from build123d import *

# Parameters (mm, degrees)
BOSS_EXTRUDE1_DEPTH = 25.1714


with BuildPart() as part:
    # Sketch1 → Boss-Extrude1 (new body)
    with BuildSketch(Plane.XY.offset(12.5857)):
        with BuildLine():
            Line((-15.096819971, 70.27139515), (-15.096819971, -8.74510913))
            ThreePointArc((-15.096819971, -8.74510913), (-13.34429465, -12.976079529), (-9.113324251, -14.72860485))
            Line((-9.113324251, -14.72860485), (9.113324251, -14.72860485))
            ThreePointArc((9.113324251, -14.72860485), (13.34429465, -12.976079529), (15.096819971, -8.74510913))
            Line((15.096819971, -8.74510913), (15.096819971, 70.27139515))
            Line((15.096819971, 70.27139515), (-15.096819971, 70.27139515))
        make_face()
    extrude(amount=-BOSS_EXTRUDE1_DEPTH)

    # Sketch2 → Revolve1 (revolve)
    with BuildSketch(Plane(origin=(0, 0, 0), x_dir=(1, 0, 0), z_dir=(0, 1, 0))):
        with BuildLine():
            Line((15.767676296, 28.0797), (0.740743286, 28.0797))
            Line((0.740743286, 28.0797), (0.740743286, 12.5857))
            Line((0.740743286, 12.5857), (10.306676296, 12.5857))
            Line((10.306676296, 12.5857), (10.306676296, 23.56842946))
            Line((10.306676296, 23.56842946), (14.543986539, 24.703813318))
            ThreePointArc((14.543986539, 24.703813318), (15.426502661, 25.293491738), (15.767676296, 26.298556857))
            Line((15.767676296, 26.298556857), (15.767676296, 28.0797))
        make_face()
    revolve(axis=Axis((0.740743286, 0, -28.0797), (0, 0, 1)))

    # Sketch3 → Revolve2 (revolve)
    with BuildSketch(Plane(origin=(0, 0, 0), x_dir=(1, 0, 0), z_dir=(0, 1, 0))):
        with BuildLine():
            Line((9.525, -12.5857), (0, -12.5857))
            Line((0, -12.5857), (0, -28.0797))
            Line((0, -28.0797), (14.986, -28.0797))
            Line((14.986, -28.0797), (14.986, -26.20110633))
            ThreePointArc((14.986, -26.20110633), (14.671070491, -25.273353912), (13.856440225, -24.72903537))
            Line((13.856440225, -24.72903537), (9.525, -23.56842946))
            Line((9.525, -23.56842946), (9.525, -12.5857))
        make_face()
    revolve(axis=Axis((0, 0, 3.0607), (0, 0, 1)))

    # Sketch4 → Cut-Revolve1 (revolve, cut)
    with BuildSketch(Plane.XZ):
        Polygon((8.636, 37.6047), (0, 37.6047), (0, -37.6047), (8.636, -37.6047), (8.636, -35.0647), (7.9375, -35.0647), (7.9375, 35.0647), (8.636, 35.0647), align=None)
    revolve(axis=Axis((0, 0, 37.6047), (0, 0, -1)), mode=Mode.SUBTRACT)


solid = part.part
Design review of the part built by this model. Coordinates are the model's own, in mm. A direction names the side the tool comes from. Round coordinates to 2 decimals unless told otherwise and drop trailing zeros. Loops run counter-clockwise (first coordinate to the right, second up) from the corner with the lowest first, then second, coordinate; pieces in that order, holes last. Notation, with made-up numbers: (-29, 59.5) -> (-23, 59.5) arc R18 cw to (-23, 80.5) -> close; hole circle Ø2 at (16, 19). An arc over 180 degrees is marked (long way). Use one line per item in the form item = value. Start each with the question number.
Q1. We need section B-B on z = -7.5. Give the boundary of the cut face in (x, y) (1 decimal).
Q2. For pin 1 Ø18.5 at (x, y) = (0, 0) entering from -Z; pin 2 Ø1 at (x, y) = (6, 20) entering from +Z; pin 3 Ø1 at (x, z) = (9, -0.5) entering from -Y; pin 4 Ø20 at (y, z) = (31.5, -5.5) entering from +X, all flat-tipped, find the tip position at first contact; note any pin that passes through.
Q3. Wall thickness on line 1 along Y through (x, z) = (0, -6); line 2 along Y through (x, z) = (0, 15) (1 decimal); line 3 along Z through (x, y) = (-4, -10.5): over which ranges is each line inside the solid? List them lowest first. Write a range as [from, to].
Q4. Draft analysis for pull direction Z (two halves, no side actions). For faces 6 (the face through (14.62, -5.76, -27.2)), 7 (the face through (-8.816, 0.421, -18.154)), 8 (the face through (7, -6, -28.08)), 9 (the face through (0, 28, -12.586)), state which applies: +Z half, -Z half, draft (parallel to the pull), parting line (faces both ways), or undercut.
Q5. We need section C-C on z = -16. Give the boundary of the cut face in (x, y) (1 decimal).
Q6. Machinability: for faces 1 (the face through (0, -14.729, 0)), 2 (the face through (-1.72, 7.75, 0.39)), 3 (the face through (-1.95, 14.86, 27.13)), 4 (the face through (-7.559, -5.796, 18)), 5 (the face through (13.3, -13.02, 0.18)), which of the approach directions +Z, -Z, +X, -X, +Y, -Y give a long, thin tool a straight path to every point of the face, cutting with its end or side? Answer none if there is none.
Q7. We need section A-A on y = 0. Give the boundary of the cut face in (x, z) (1 decimal).
Calculated:
q1.outline = (-15.1, -8.7) arc R6 ccw to (-9.1, -14.7) -> (9.1, -14.7) arc R6 ccw to (15.1, -8.7) -> (15.1, 70.3) -> (-15.1, 70.3) -> close; hole circle Ø15.9 at (0, 0)
q2.pin_1 = -28.08
q2.pin_2 = 12.59
q2.pin_3 = -14.73
q2.pin_4 = 15.1
q3.line_1 = [-14.73, -7.94], [7.94, 70.27]
q3.line_2 = [-9.5, -7.9], [7.9, 9.5]
q3.line_3 = [-28.08, -24.09], [-12.59, 12.59], [24.03, 28.08]
q4.face_6 = draft
q4.face_7 = undercut
q4.face_8 = -Z half
q4.face_9 = undercut
q5.outline = circle Ø19.1 at (0.7, 0); hole circle Ø15.9 at (0, 0)
q6.face_1 = +X, -X, -Y
q6.face_2 = +Z, -Z
q6.face_3 = +Z
q6.face_4 = none
q6.face_5 = +Z, -Z, +X, -Y
q7.outline = (-15.1, -12.6) -> (-8.8, -12.6) -> (-8.8, -23.6) -> (-13.1, -24.7) arc R1.7 ccw to (-14.3, -26.3) -> (-14.3, -28.1) -> (-7.9, -28.1) -> (-7.9, 28.1) -> (-15, 28.1) -> (-15, 26.2) arc R1.5 ccw to (-13.9, 24.7) -> (-9.5, 23.6) -> (-9.5, 12.6) -> (-15.1, 12.6) -> close; (7.9, -28.1) -> (15.8, -28.1) -> (15.8, -26.3) arc R1.7 ccw to (14.5, -24.7) -> (10.3, -23.6) -> (10.3, -12.6) -> (15.1, -12.6) -> (15.1, 12.6) -> (9.5, 12.6) -> (9.5, 23.6) -> (13.9, 24.7) arc R1.5 ccw to (15, 26.2) -> (15, 28.1) -> (7.9, 28.1) -> close
